from build123d import *

# Parameters (mm, degrees)
ESQUISSE1_R             = 47.5
BOSS_EXTRU_1_DEPTH      = 6
ESQUISSE9_W             = 150
ESQUISSE9_H             = 120
BOSS_EXTRU_2_DEPTH      = 10
ESQUISSE10_W            = 6
ESQUISSE10_H            = 50
ESQUISSE10_W_2          = 50
ESQUISSE10_H_2          = 6
ENL_V_MAT_EXTRU_1_DEPTH = 10
ESQUISSE11_W            = 670.254020464
ESQUISSE11_H            = 265.771999275
ENL_V_MAT_EXTRU_2_DEPTH = 10
ESQUISSE12_R            = 2.5
ENL_V_MAT_EXTRU_3_DEPTH = 10


with BuildPart() as part:
    # Esquisse1 → Boss.-Extru.1 (new body)
    with BuildSketch(Plane.XY):
        Polygon((-255.775862069, 10.959681362), (-205, -75.190256718), (205, -75.190256718), (255.775862069, 10.959681362), (50, 336.353741833), (-50, 336.353741833), align=None)
        with Locations((-157.5, 0)):
            Circle(ESQUISSE1_R, mode=Mode.SUBTRACT)
        with Locations((-52.5, 0)):
            Circle(ESQUISSE1_R, mode=Mode.SUBTRACT)
        with Locations((52.5, 0)):
            Circle(ESQUISSE1_R, mode=Mode.SUBTRACT)
        with Locations((157.5, 0)):
            Circle(ESQUISSE1_R, mode=Mode.SUBTRACT)
        with Locations((-105, 90.932667397)):
            Circle(ESQUISSE1_R, mode=Mode.SUBTRACT)
        with Locations((0, 90.932667397)):
            Circle(ESQUISSE1_R, mode=Mode.SUBTRACT)
        with Locations((105, 90.932667397)):
            Circle(ESQUISSE1_R, mode=Mode.SUBTRACT)
        with Locations((-52.5, 181.865334795)):
            Circle(ESQUISSE1_R, mode=Mode.SUBTRACT)
        with Locations((52.5, 181.865334795)):
            Circle(ESQUISSE1_R, mode=Mode.SUBTRACT)
        with Locations((0, 272.798002192)):
            Circle(ESQUISSE1_R, mode=Mode.SUBTRACT)
    extrude(amount=BOSS_EXTRU_1_DEPTH)

    # Esquisse9 → Boss.-Extru.2 (add)
    with BuildSketch(Plane.XY.offset(6)):
        with Locations((0, -135.190256718)):
            Rectangle(ESQUISSE9_W, ESQUISSE9_H)
    extrude(amount=-BOSS_EXTRU_2_DEPTH)

    # Esquisse10 → Enlèv. mat.-Extru.1 (cut)
    with BuildSketch(Plane.XY.offset(6)):
        with Locations((-72, -129.244737692)):
            Rectangle(ESQUISSE10_W, ESQUISSE10_H)
        with Locations((0, -192.190256718)):
            Rectangle(ESQUISSE10_W_2, ESQUISSE10_H_2)
        with Locations((-140, -72.190256718)):
            Rectangle(ESQUISSE10_W_2, ESQUISSE10_H_2)
        Polygon((-217.693965517, -53.652772198), (-212.524969232, -50.606220473), (-237.912900267, -7.531251434), (-243.081896552, -10.577803158), align=None)
        Polygon((-229.051724138, 53.218650255), (-223.980647871, 50.011753703), (-170.532372009, 134.529691487), (-175.603448276, 137.736588039), align=None)
        Polygon((-130.172413793, 209.576835156), (-125.101337526, 206.369938604), (-71.653061664, 290.887876389), (-76.724137931, 294.094772941), align=None)
        with Locations((0, 333.353741833)):
            Rectangle(ESQUISSE10_W_2, ESQUISSE10_H_2)
        Polygon((71.653061664, 290.887876389), (76.724137931, 294.094772941), (130.172413793, 209.576835156), (125.101337526, 206.369938604), align=None)
        Polygon((170.532372009, 134.529691487), (175.603448276, 137.736588039), (229.051724138, 53.218650255), (223.980647871, 50.011753703), align=None)
        Polygon((237.912900267, -7.531251434), (243.081896552, -10.577803158), (217.693965517, -53.652772198), (212.524969232, -50.606220473), align=None)
        with Locations((140, -72.190256718)):
            Rectangle(ESQUISSE10_W_2, ESQUISSE10_H_2)
        with Locations((72, -129.244737692)):
            Rectangle(ESQUISSE10_W, ESQUISSE10_H)
    extrude(amount=-ENL_V_MAT_EXTRU_1_DEPTH, mode=Mode.SUBTRACT)

    # Esquisse11 → Enlèv. mat.-Extru.2 (cut)
    with BuildSketch(Plane.XY.offset(6)):
        with Locations((-20.35830969, -62.304257081)):
            Rectangle(ESQUISSE11_W, ESQUISSE11_H)
    extrude(amount=-ENL_V_MAT_EXTRU_2_DEPTH, mode=Mode.SUBTRACT)

    # Esquisse12 → Enlèv. mat.-Extru.3 (cut)
    with BuildSketch(Plane.XY.offset(6)):
        with Locations((-52.5, 126.865334795)):
            Circle(ESQUISSE12_R)
        with Locations((52.5, 126.865334795)):
            Circle(ESQUISSE12_R)
        with Locations((0, 217.798002192)):
            Circle(ESQUISSE12_R)
    extrude(amount=-ENL_V_MAT_EXTRU_3_DEPTH, mode=Mode.SUBTRACT)


solid = part.part
Source: CAD feature listing. Evaluate the final solid. Frame: model axes, mm. Coordinates: 2 decimals unless noted, no trailing zeros. Loops run counter-clockwise (first coordinate to the right, second up) from the corner with the lowest first, then second, coordinate; pieces in that order, holes last. Notation, with made-up numbers: (-17, -13.5) -> (16, -13.5) arc R19 cw to (16, -7.5) -> close; hole circle Ø5 at (-38.75, 82). An arc over 180 degrees is marked (long way). Answer in a Markdown table with one row per item. Add a question column.
Q1. Section C-C on z = 3.75. Give the number of separate pieces and of enclosed holes in the cut face, and give its area (3 significant figures).
Q2. Section D-D on x = 105. Return the cut outline in (y, z), and give its area (3 significant figures).
Q3. Pull-direction query (Y, two-part tool) for faces 1 (the face through (63.55, 314.93, 2.96)), 2 (the face through (-1, 184, 0)), 3 (the face through (1.339, 138.414, 2.958)); classes: pulls with the +Y half, pulls with the -Y half, needs draft (parallel to the pull), parting line crosses it, or undercut.
Q4. Contact query for flat-ended pins moving along their axis: pin 1 Ø1.8 at (y, z) = (333.5, 3) entering from +X; pin 2 Ø8 at (x, y) = (52.5, 126.87) entering from +Z; pin 3 Ø1.5 at (y, z) = (220, 3.5) entering from +X; pin 4 Ø1 at (y, z) = (164.5, 5) entering from +X. Output: stop coordinate, or through.
Q5. Section A-A on y = 286.5. Return the cut outline in (x, z).
Q6. Ray query, line 1 along Y through (x, z) = (0, 1.6); line 2 along X through (y, z) = (178.5, 4); line 3 along X through (y, z) = (198, 1.75). Return the intervals inside material, ascending.
Q7. Section B-B on x = 35. Return the cut outline in (y, z).
Computed values:
| question | item | result |
|---|---|---|
| 1 | separate pieces | 1 |
| 1 | enclosed holes | 6 |
| 1 | area | 31,200 mm^2 |
| 2 | outline | (138.43, 0) -> (238.16, 0) -> (238.16, 6) -> (138.43, 6) -> close |
| 2 | area | 598 mm^2 |
| 3 | face 1 | pulls with the +Y half |
| 3 | face 2 | needs draft |
| 3 | face 3 | undercut |
| 4 | pin 1 | stops at x = 52.37 |
| 4 | pin 2 | stops at z = 6 |
| 4 | pin 3 | stops at x = 116.96 |
| 4 | pin 4 | stops at x = 158.99 |
| 5 | outline | (-74.43, 0) -> (-45.48, 0) -> (-45.48, 6) -> (-74.43, 6) -> close; (45.48, 0) -> (74.43, 0) -> (74.43, 6) -> (45.48, 6) -> close |
| 6 | line 1 | y = 138.43 to 215.3, 220.3 to 225.3, 320.3 to 330.35 |
| 6 | line 2 | x = -149.83 to -99.88, -5.12 to 5.12, 99.88 to 149.83 |
| 6 | line 3 | x = -137.49 to -97.18, -7.82 to 7.82, 97.18 to 137.49 |
| 7 | outline | (123.05, 0) -> (137.71, 0) -> (137.71, 6) -> (123.05, 6) -> close; (226.02, 0) -> (240.68, 0) -> (240.68, 6) -> (226.02, 6) -> close; (304.91, 0) -> (336.35, 0) -> (336.35, 6) -> (304.91, 6) -> close |
